Design review of the part shown in the three views and the two pictorial views. Dimensions are in mm from the part's minimum x, y and z. Round coordinates to 2 decimals unless told otherwise and drop trailing zeros. Write each loop counter-clockwise with the first axis right and the second up, starting at its lowest first coordinate (ties: lowest second). Pieces come first, ordered by that corner, then holes. Notation, with made-up numbers: (-12, 12) -> (30, 12) arc R31 cw to (30, 49) -> close; hole circle Ø1 at (-30, 16). An arc over 180 degrees is marked (long way). Answer as a JSON object with one key per item and string values. Group by question number.
1) To check wall thickness, follow probe 1 along X at (y, z) = (8.25, 0.6); probe 2 along Y at (x, z) = (9, 1.35); probe 3 along X at (y, z) = (5.5, 4.35). State the ranges of each line that lie inside material, in increasing order. Write a range as [from, to].
2) Mouldability with a two-part tool opening along X and no side actions: class the marked faces 1, 2 and 3 as pulls with the +X half, pulls with the -X half, needs draft (parallel to the pull), parting line crosses it, or undercut.
3) Insertion check: pin 1 Ø3 at (x, y) = (2.5, 11) entering from -Z; pin 2 Ø2 at (x, y) = (10.5, 7) entering from +Z. Each pin has a flat end and moves straight along its axis. Give the tip position at first contact, or say it passes through.
4) We need section A-A, the plane z = 1.6. Write out the cut boundary in (x, y) (3 decimals).
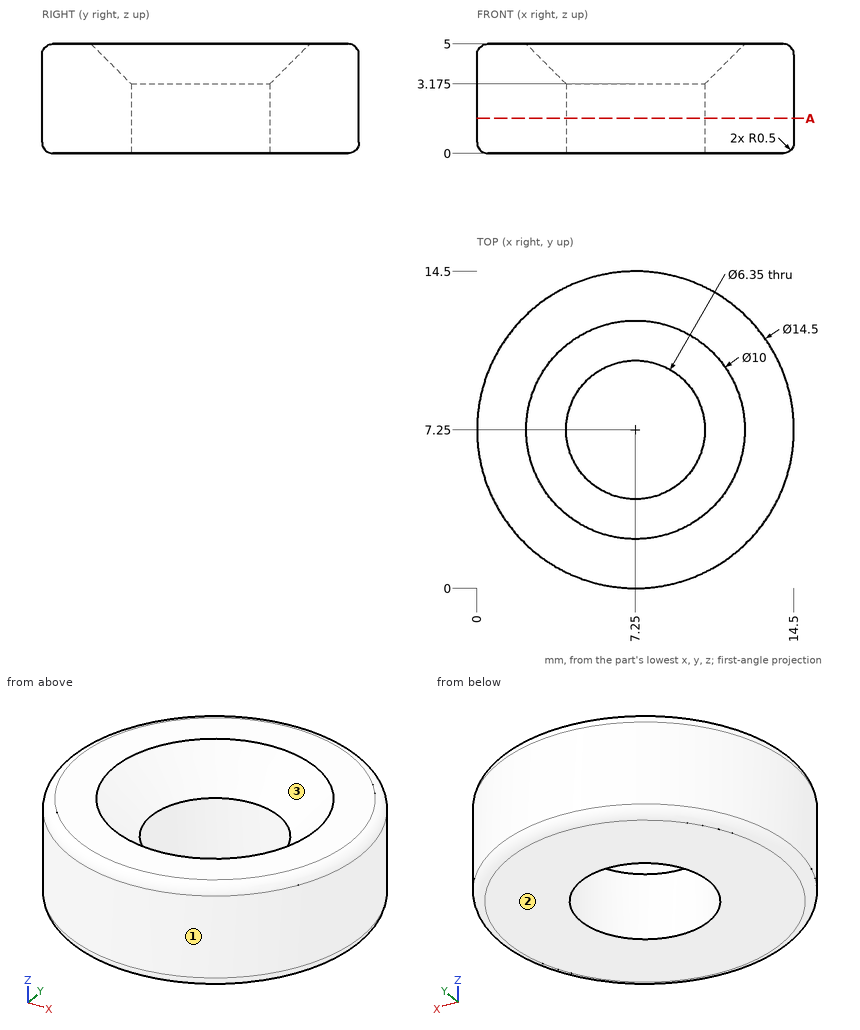
Here are the results:
{
 "1": {"probe 1": "x = [0.07, 4.24], [10.26, 14.43]", "probe 2": "y = [0.21, 4.6], [9.9, 14.29]", "probe 3": "x = [0.21, 3.27], [11.23, 14.29]"},
 "2": {"face 1": "parting line crosses it", "face 2": "needs draft", "face 3": "undercut"},
 "3": {"pin 1": "stops at z = 0", "pin 2": "stops at z = 4.26"},
 "4": {"outline": "circle Ø14.5 at (7.25, 7.25); hole circle Ø6.35 at (7.25, 7.25)"}
}
